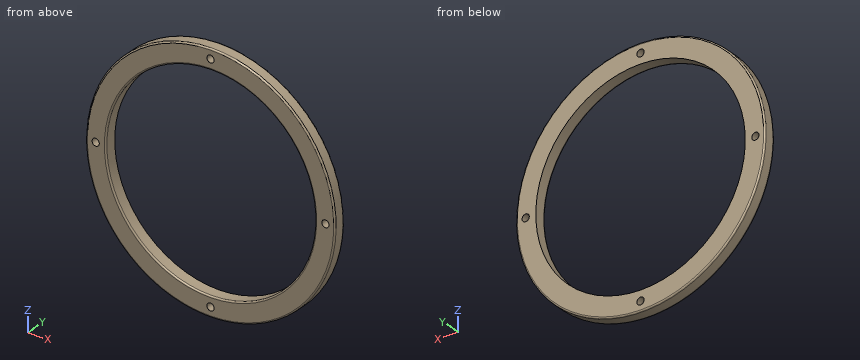
from build123d import *

# Parameters (mm, degrees)
SKETCH1_R           = 86.25
SKETCH1_R_2         = 72.5
BOSS_EXTRUDE1_DEPTH = 8.5
FILLET1_R           = 1
M6_TAPPED_HOLE1_D   = 5


with BuildPart() as part:
    # Sketch1 → Boss-Extrude1 (new body)
    with BuildSketch(Plane(origin=(0, 0, 0), x_dir=(1, 0, 0), z_dir=(0, 1, 0))):
        with Locations(Location((0, 0, 0), (0, 0, 270))):
            Circle(SKETCH1_R)
        with Locations(Location((0, 0, 0), (0, 0, 270))):
            Circle(SKETCH1_R_2, mode=Mode.SUBTRACT)
    extrude(amount=BOSS_EXTRUDE1_DEPTH)

    # Fillet1
    fillet1_edges = [part.edges().sort_by_distance(p)[0] for p in [
        (0, 0, -86.25),
        (0, 8.5, -86.25),
        (0, 0, -72.5),
    ]]
    fillet(fillet1_edges, radius=FILLET1_R)

    # M6 Tapped Hole1 (through all)
    with Locations(Plane(origin=(0, 8.5, 0), x_dir=(1, 0, 0), z_dir=(0, 1, 0))):
        with Locations((0, 79.5), (79.5, 0), (0, -79.5), (-79.5, 0)):
            Hole(M6_TAPPED_HOLE1_D / 2)


solid = part.part
Design review of the part built by this model. Coordinates are the model's own, in mm. Coordinates: 2 decimals unless noted, no trailing zeros. Write each loop counter-clockwise with the first axis right and the second up, starting at its lowest first coordinate (ties: lowest second). Pieces come first, ordered by that corner, then holes. Notation, with made-up numbers: (-7.5, 7.25) -> (1.5, 7.25) arc R16 ccw to (1.5, 37.25) -> close; hole circle Ø9 at (83.25, 57). An arc over 180 degrees is marked (long way). Write each question's results on one line, items separated by ' | '. Start each with the question number.
(1) Clearance check with flat-ended pins moving along their axes: P1, Ø2, axis at x = 34, y = 4, coming from the +Z side; P2, Ø4, axis at x = 35, y = 3.5, coming from the -Z side. State where each tip first meets the part, or that it passes through.
(2) Take a section at B-B on y = 4.25. Write out the cut boundary in (x, z).
(3) For line 1 along Z through (x, y) = (-66.5, 5.75); line 2 along Z through (x, y) = (-30, 3.5); line 3 along X through (y, z) = (5.5, 40), list the stretches that pass through material, from the lowest coordinate up. Write a range as from..to.
(4) Take a section at A-A on x = 0. Write out the cut boundary in (y, z), and give its area (3 significant figures).
Results found:
1) P1: stops at z = 79.69 | P2: stops at z = -79.69
2) outline: circle Ø172.5 at (0, 0); hole circle Ø5 at (-79.5, 0); hole circle Ø145 at (0, 0); hole circle Ø5 at (0, -79.5); hole circle Ø5 at (0, 79.5); hole circle Ø5 at (79.5, 0)
3) line 1: z = -54.93..-28.88, 28.88..54.93 | line 2: z = -80.86..-66, 66..80.86 | line 3: x = -76.41..-60.47, 60.47..76.41
4) outline: (0, -85.25) arc R1 ccw to (1, -86.25) -> (7.5, -86.25) arc R1 ccw to (8.5, -85.25) -> (8.5, -82) -> (0, -82) -> close; (0, -77) -> (8.5, -77) -> (8.5, -72.5) -> (1, -72.5) arc R1 ccw to (0, -73.5) -> close; (0, 73.5) arc R1 ccw to (1, 72.5) -> (8.5, 72.5) -> (8.5, 77) -> (0, 77) -> close; (0, 82) -> (8.5, 82) -> (8.5, 85.25) arc R1 ccw to (7.5, 86.25) -> (1, 86.25) arc R1 ccw to (0, 85.25) -> close | area: 147 mm2
